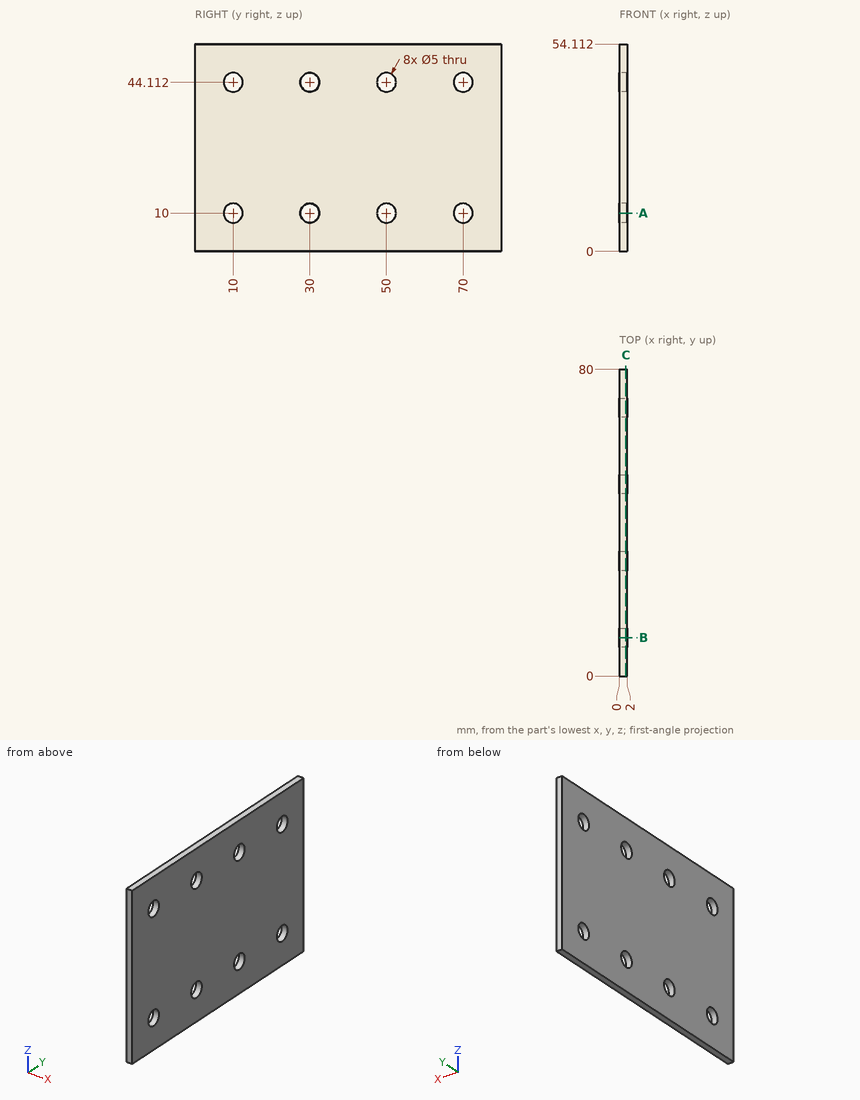
Print and shaded views of the part. All mm, measured from the part's lowest x, y and z. Give positions to 0.01 mm unless a question says otherwise; leave off trailing zeros. Loops run counter-clockwise (first coordinate to the right, second up) from the corner with the lowest first, then second, coordinate; pieces in that order, holes last. Notation, with made-up numbers: (14, -13) -> (70, -13) arc R14 cw to (70, 3) -> close; hole circle Ø5 at (26.5, -3). An arc over 180 degrees is marked (long way). Use a Markdown table: item, result.
1. Wall check: L1, parallel to Z at x = 0.7, y = 50; L2, parallel to Y at x = 1.1, z = 9.5. Give the ranges that are in metal, low to high. Write a range as [from, to].
Check result:
| item | result |
|---|---|
| L1 | z = [0, 7.5], [12.5, 41.61], [46.61, 54.11] |
| L2 | y = [0, 7.55], [12.45, 27.55], [32.45, 47.55], [52.45, 67.55], [72.45, 80] |
2. Slice it at B-B (y = 10). List the corners of the cut face in (x, z).
Check result:
| item | result |
|---|---|
| outline | (0, 0) -> (2, 0) -> (2, 7.5) -> (0, 7.5) -> close; (0, 12.5) -> (2, 12.5) -> (2, 41.61) -> (0, 41.61) -> close; (0, 46.61) -> (2, 46.61) -> (2, 54.11) -> (0, 54.11) -> close |
3. Slice it at C-C (x = 1.65). Give the number of separate pieces and of enclosed holes in the cut face, plus the area to 3 significant figures.
Check result:
| item | result |
|---|---|
| separate pieces | 1 |
| enclosed holes | 8 |
| area | 4,170 mm^2 |
4. Flat gauge pin, fed straight in: pin 1 (4.5 mm diameter, centred on y = 30, z = 44.112, fed in from -X). Where does the tip first touch, or does it go through?
Check result:
| item | result |
|---|---|
| pin 1 | passes through |
5. Slice it at A-A (z = 10). List the corners of the cut face in (x, y).
Check result:
| item | result |
|---|---|
| outline | (0, 0) -> (2, 0) -> (2, 7.5) -> (0, 7.5) -> close; (0, 12.5) -> (2, 12.5) -> (2, 27.5) -> (0, 27.5) -> close; (0, 32.5) -> (2, 32.5) -> (2, 47.5) -> (0, 47.5) -> close; (0, 52.5) -> (2, 52.5) -> (2, 67.5) -> (0, 67.5) -> close; (0, 72.5) -> (2, 72.5) -> (2, 80) -> (0, 80) -> close |
